Print and shaded views of the part. All mm, measured from the part's lowest x, y and z. A direction names the side the tool comes from. Coordinates: 2 decimals unless noted, no trailing zeros. Loops run counter-clockwise (first coordinate to the right, second up) from the corner with the lowest first, then second, coordinate; pieces in that order, holes last. Notation, with made-up numbers: (40, -36) -> (73, -36) arc R17 cw to (73, -8) -> close; hole circle Ø4 at (-8.5, -5.5). An arc over 180 degrees is marked (long way). One line per item, written item: value. Start each with the question number.
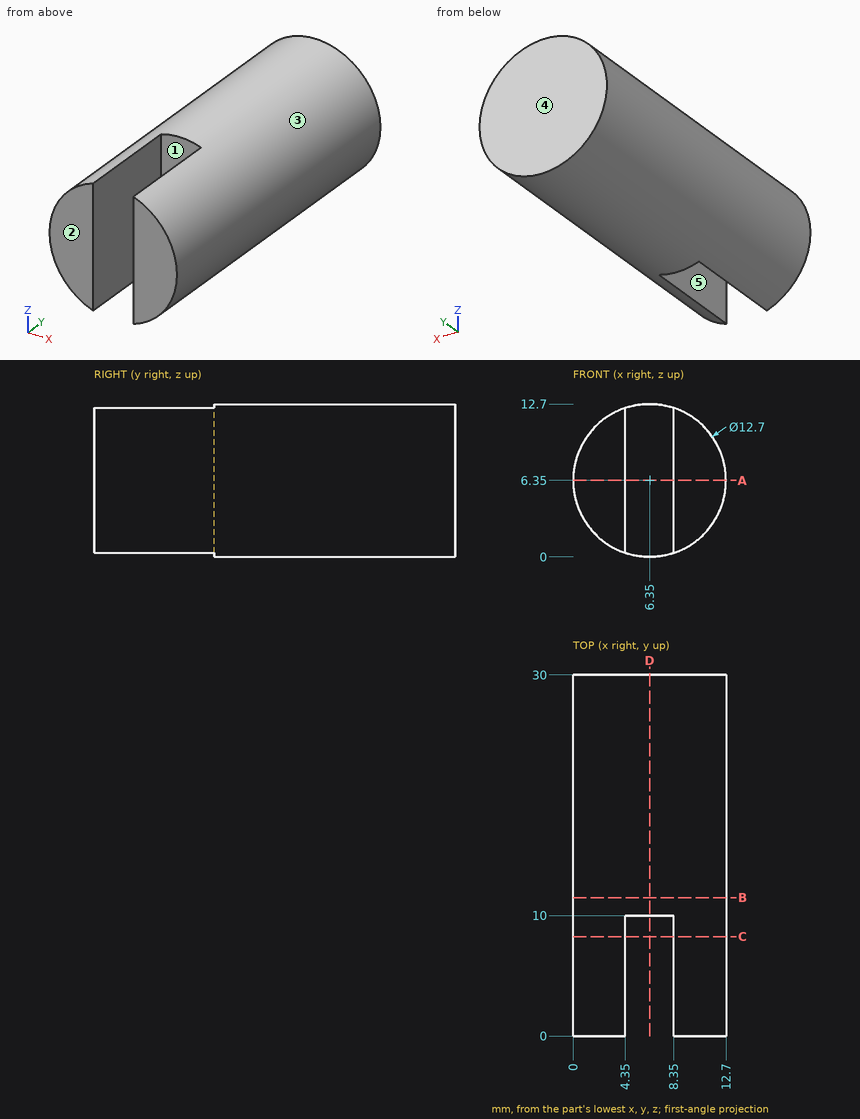
1) Tool access for the marked faces 4 and 5: list every direction of +Z, -Z, +X, -X, +Y, -Y with a clear straight run to the whole face (end or side of a thin tool).
2) Pin check, flat tips, straight feed: pin 1 Ø1 at (x, z) = (6, 7.5) entering from -Y; pin 2 Ø1 at (x, y) = (2, 6) entering from -Z; pin 3 Ø6 at (x, y) = (2, 4) entering from +Z. Stop position of each tip, or through.
3) Slice it at C-C (y = 8.25). Give the cut face in (x, z).
4) Probe line 1 (Y direction, x = 8, z = 2.25); line 2 (X direction, y = 7, z = 2.25); line 3 (X direction, y = 20, z = 6.5). List the from-to ranges inside material, lowest first. Write a range as from..to.
5) Slice it at A-A (z = 6.35). Give the cut face in (x, y), then the cut area to 3 significant figures.
6) Slice it at B-B (y = 11.5). Give the cut face in (x, z), then the cut area to 3 significant figures.
7) Slice it at D-D (x = 6.35). Give the cut face in (y, z), then the cut area to 3 significant figures.
8) Pull direction X, two halves, no side cores. Call the marked faces 1, 2 and 3: +X half, -X half, draft (parallel to the pull), parting line (faces both ways), or undercut.
Check sheet entries:
1. face 4: +Z, -Z, +X, -X, +Y
1. face 5: +Z, -Z, -Y
2. pin 1: stops at y = 10
2. pin 2: stops at z = 1.3
2. pin 3: stops at z = 12.38
3. outline: (4.35, 0.32) -> (4.35, 12.38) arc R6.35 ccw to start; (8.35, 0.32) arc R6.35 ccw to (8.35, 12.38) -> close
4. line 1: y = 10..30
4. line 2: x = 1.5..4.35, 8.35..11.2
4. line 3: x = 0..12.7
5. outline: (0, 0) -> (4.35, 0) -> (4.35, 10) -> (8.35, 10) -> (8.35, 0) -> (12.7, 0) -> (12.7, 30) -> (0, 30) -> close
5. area: 341 mm^2
6. outline: circle Ø12.7 at (6.35, 6.35)
6. area: 127 mm^2
7. outline: (10, 0) -> (30, 0) -> (30, 12.7) -> (10, 12.7) -> close
7. area: 254 mm^2
8. face 1: undercut
8. face 2: draft
8. face 3: parting line
